Work out the finished part from the listing and answer in its coordinate system (mm). Face numbers are marked on the shaded views. Round coordinates to 2 decimals unless told otherwise and drop trailing zeros. Write each loop counter-clockwise with the first axis right and the second up, starting at its lowest first coordinate (ties: lowest second). Pieces come first, ordered by that corner, then holes. Notation, with made-up numbers: (-9.5, -24.5) -> (8.5, -24.5) arc R17 ccw to (8.5, -2.5) -> close; hole circle Ø2 at (3.5, 22.25). An arc over 180 degrees is marked (long way). Answer as a JSON object with one key per item and string values. Group by question number.
from build123d import *

# Parameters (mm, degrees)
SKETCH1_R           = 35
SKETCH1_R_2         = 1.65
SKETCH1_R_3         = 1.5
SKETCH1_R_4         = 2.5
BOSS_EXTRUDE1_DEPTH = 5


with BuildPart() as part:
    # Sketch1 → Boss-Extrude1 (new body)
    with BuildSketch(Plane.XY):
        Circle(SKETCH1_R)
        with Locations((0, 25)):
            Circle(SKETCH1_R_2, mode=Mode.SUBTRACT)
        with Locations((21.650635095, -12.5)):
            Circle(SKETCH1_R_2, mode=Mode.SUBTRACT)
        with Locations((-21.650635095, -12.5)):
            Circle(SKETCH1_R_2, mode=Mode.SUBTRACT)
        Circle(SKETCH1_R_3, mode=Mode.SUBTRACT)
        with Locations((0, 7)):
            Circle(SKETCH1_R_4, mode=Mode.SUBTRACT)
        with Locations((6.062177826, 3.5)):
            Circle(SKETCH1_R_4, mode=Mode.SUBTRACT)
        with Locations((6.062177826, -3.5)):
            Circle(SKETCH1_R_4, mode=Mode.SUBTRACT)
        with Locations((0, -7)):
            Circle(SKETCH1_R_4, mode=Mode.SUBTRACT)
        with Locations((-6.062177826, -3.5)):
            Circle(SKETCH1_R_4, mode=Mode.SUBTRACT)
        with Locations((-6.062177826, 3.5)):
            Circle(SKETCH1_R_4, mode=Mode.SUBTRACT)
    extrude(amount=BOSS_EXTRUDE1_DEPTH)


solid = part.part
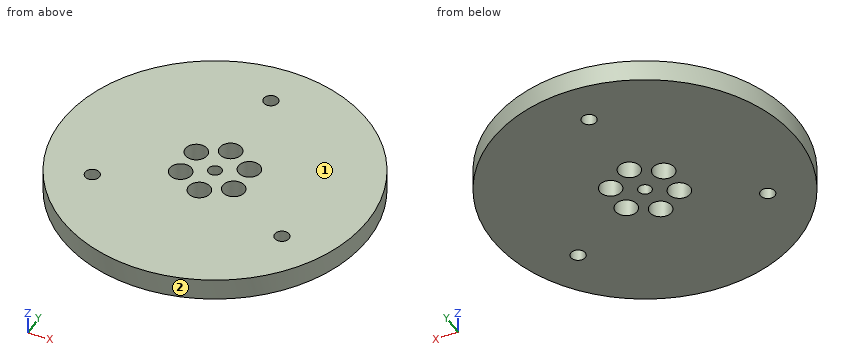
1) A cutting plane is placed at B-B on y = 0. Determine the outline of the cut face in (x, z).
2) A cutting plane is placed at D-D on y = -12.5. Determine the outline of the cut face in (x, z), plus the area to 3 significant figures.
3) For a pull along X with two mould halves and no side action, classify the marked faces 1 and 2 as released by +X, released by -X, zero draft, split by the parting line, or undercut.
4) A cutting plane is placed at A-A on z = 2.3. State how many separate pieces and enclosed holes the cut face has, plus the area to 3 significant figures.
5) Straight lines are drawn through the part: L1, parallel to Y at x = 0, z = 1.5; L2, parallel to Y at x = 4, z = 1.75; L3, parallel to X at y = 18, z = 2.85. For each, find the intervals that lie inside material, in ascending order.
6) This flat-tipped pin is pushed along its axis until it touches: P1, Ø2, axis at x = -0.5, z = 1, coming from the -Y side. Where does it stop, or does it pass through?
7) A cutting plane is placed at C-C on x = -4.5. Determine the outline of the cut face in (y, z).
Established:
{
 "1": {"outline": "(-35, 0) -> (-1.5, 0) -> (-1.5, 5) -> (-35, 5) -> close; (1.5, 0) -> (35, 0) -> (35, 5) -> (1.5, 5) -> close"},
 "2": {"outline": "(-32.69, 0) -> (-23.3, 0) -> (-23.3, 5) -> (-32.69, 5) -> close; (-20, 0) -> (20, 0) -> (20, 5) -> (-20, 5) -> close; (23.3, 0) -> (32.69, 0) -> (32.69, 5) -> (23.3, 5) -> close", "area": "294 mm²"},
 "3": {"face 1": "zero draft", "face 2": "split by the parting line"},
 "4": {"separate pieces": "1", "enclosed holes": "10", "area": "3,700 mm²"},
 "5": {"L1": "y = -35 to -9.5, -4.5 to -1.5, 1.5 to 4.5, 9.5 to 23.35, 26.65 to 35", "L2": "y = -34.77 to -4.91, -2.09 to 2.09, 4.91 to 34.77", "L3": "x = -30.02 to 30.02"},
 "6": {"P1": "stops at y = -35"},
 "7": {"outline": "(-34.71, 0) -> (-5.45, 0) -> (-5.45, 5) -> (-34.71, 5) -> close; (-1.55, 0) -> (1.55, 0) -> (1.55, 5) -> (-1.55, 5) -> close; (5.45, 0) -> (34.71, 0) -> (34.71, 5) -> (5.45, 5) -> close"}
}
